Build history of the part. All positions in model axes, mm. A direction names the side the tool comes from. Give positions to 0.01 mm unless a question says otherwise; leave off trailing zeros. Answer as a JSON object with one key per item and string values. Group by question number.
Q1. Drop flat-ended pins along their axis: pin 1 (5 mm diameter, centred on x = -6.5, z = -1.5, fed in from +Y); pin 2 (5 mm diameter, centred on x = -4, z = -15.5, fed in from +Y); pin 3 (4 mm diameter, centred on x = -4.95, z = 4.95, fed in from -Y); pin 4 (1.8 mm diameter, centred on x = 10.45, z = -4, fed in from +Y). Give the stop position or say it passes through.
Q2. Wall check: probe 1 along X at (y, z) = (0.85, 4); probe 2 along Z at (x, y) = (6, 8.75); probe 3 along Z at (x, y) = (-6.25, 7.5). Give the ranges that are in metal, low to high. Write a range as from..to.
Q3. Two-plate mould, pull along X, no slides. Class faces 5 (the flat face through (8.5, 9, 0)), 6 (the cylindrical face through (0.13, 8.97, -13.25)), 7 (the cylindrical face through (-0.14, 10.49, -10.25)), 8 (the flat face through (0, 7, -20)): pulls with the +X half, pulls with the -X half, needs draft (parallel to the pull), parting line crosses it, or undercut.
Q4. Band-saw the part on A-A, the plane y = 1.25. Count the separate pieces of the cut face and the enclosed holes in it, plus the area to 3 significant figures.
Q5. Tool access for faces 1 (the cylindrical face through (-8.814, 4.163, -4.215)), 2 (the flat face through (-0.1, 11, -10.4)), 3 (the cylindrical face through (7.924, 4.327, -5.34)), 4 (the flat face through (-6.44, 1.01, -0.05)): list every direction of +Z, -Z, +X, -X, +Y, -Y with a clear straight run to the whole face (end or side of a thin tool).
from build123d import *

# Parameters (mm, degrees)
SKETCH1_W           = 25
SKETCH1_H           = 52
BOSS_EXTRUDE1_DEPTH = 7
SKETCH2_R           = 1
CUT_EXTRUDE1_DEPTH  = 30.685855218
LPATTERN1_COUNT     = 6
LPATTERN1_PITCH     = 8
CHAMFER2_SIZE       = 4
SKETCH10_W          = 14.9
SKETCH10_H          = 52
CUT_EXTRUDE4_DEPTH  = 2
CHAMFER3_SIZE       = 2
BOSS_EXTRUDE2_DEPTH = 3
BOSS_EXTRUDE3_DEPTH = 4
SKETCH13_R          = 1.65
CUT_EXTRUDE5_DEPTH  = 3
CUT_EXTRUDE6_REACH  = 31.686
SKETCH14_R          = 3
SKETCH16_R          = 1.65
CUT_EXTRUDE7_DEPTH  = 4.5


# Some blends are built 0.0001 mm under size
with BuildPart() as part:
    # Sketch1 → Boss-Extrude1 (new body)
    with BuildSketch(Plane(origin=(0, 0, 0), x_dir=(1, 0, 0), z_dir=(0, 1, 0))):
        Rectangle(SKETCH1_W, SKETCH1_H)
    extrude(amount=BOSS_EXTRUDE1_DEPTH)

    # Sketch2 → Cut-Extrude1 (cut, through all)
    with BuildSketch(Plane(origin=(0, 7, 0), x_dir=(1, 0, 0), z_dir=(0, 1, 0))):
        with Locations(Location((-10.45, -20, 0), (0, 0, 270))):
            Circle(SKETCH2_R)
        with Locations(Location((10.45, -20, 0), (0, 0, 270))):
            Circle(SKETCH2_R)
    cut_extrude1 = extrude(amount=-CUT_EXTRUDE1_DEPTH, mode=Mode.SUBTRACT)

    # LPattern1: Cut-Extrude1 ×6
    with Locations(*[(0, 0, -i * LPATTERN1_PITCH) for i in range(1, LPATTERN1_COUNT)]):
        add(cut_extrude1, mode=Mode.SUBTRACT)

    # Chamfer2
    # the kernel refuses this chamfer: 4 mm, written as the material it takes off along each edge
    with BuildSketch(Plane(origin=(-12.5, 7, -36.286731952), x_dir=(-0.027495876610586487, -0.9996219169112968, 0), z_dir=(0, 0, 1)), Plane(origin=(12.5, 7, 36.286731952), x_dir=(0.027495876610586487, -0.9996219169112968, 0), z_dir=(0, 0, -1))) as chamfer2_piece_1:
        Polygon((CHAMFER2_SIZE * 0.999621916911, CHAMFER2_SIZE * 0.0274958766106), (-CHAMFER2_SIZE * 0.0274958766106, CHAMFER2_SIZE * 0.999621916911), (0, 0), align=None)
    extrude(amount=72.573463904, mode=Mode.SUBTRACT)

    # Sketch10 → Cut-Extrude4 (cut)
    with BuildSketch(Plane.XZ):
        Rectangle(SKETCH10_W, SKETCH10_H)
    extrude(amount=-CUT_EXTRUDE4_DEPTH, mode=Mode.SUBTRACT)

    # Chamfer3
    chamfer3_edges = [part.edges().sort_by_distance(p)[0] for p in [
        (7.45, 2, 0),
        (-7.45, 2, 0),
    ]]
    chamfer(chamfer3_edges, length=CHAMFER3_SIZE - 0.0001)  # a hair under: the kernel refuses the full size

    # Sketch12 → Boss-Extrude2 (add)
    with BuildSketch(Plane(origin=(0, 7, 0), x_dir=(1, 0, 0), z_dir=(0, 1, 0))):
        with BuildLine():
            ThreePointArc((8.5, 5.728219619), (0, 10.25), (-8.5, 5.728219619))
            Line((-8.5, 5.728219619), (-8.5, -5.728219619))
            ThreePointArc((-8.5, -5.728219619), (0, -10.25), (8.5, -5.728219619))
            Line((8.5, -5.728219619), (8.5, 5.728219619))
        make_face()
    extrude(amount=BOSS_EXTRUDE2_DEPTH)

    # Sketch12<3> → Boss-Extrude3 (add)
    with BuildSketch(Plane(origin=(0, 7, 0), x_dir=(1, 0, 0), z_dir=(0, 1, 0))):
        with BuildLine():
            ThreePointArc((8.5, 10.164275675), (0, 13.25), (-8.5, 10.164275675))
            Line((-8.5, 10.164275675), (-8.5, 5.728219619))
            ThreePointArc((-8.5, 5.728219619), (0, 10.25), (8.5, 5.728219619))
            Line((8.5, 5.728219619), (8.5, 10.164275675))
        make_face()
        with BuildLine():
            Line((-8.5, -5.728219619), (-8.5, -10.164275675))
            ThreePointArc((-8.5, -10.164275675), (0, -13.25), (8.5, -10.164275675))
            Line((8.5, -10.164275675), (8.5, -5.728219619))
            ThreePointArc((8.5, -5.728219619), (0, -10.25), (-8.5, -5.728219619))
        make_face()
    extrude(amount=BOSS_EXTRUDE3_DEPTH)

    # Sketch13 → Cut-Extrude5 (cut)
    with BuildSketch(Plane(origin=(0, 10, 0), x_dir=(1, 0, 0), z_dir=(0, 1, 0))):
        with Locations(Location((-4.949747468, 4.949747468, 0), (0, 0, 270))):
            Circle(SKETCH13_R)
        with Locations(Location((4.949747468, 4.949747468, 0), (0, 0, 270))):
            Circle(SKETCH13_R)
        with Locations(Location((4.949747468, -4.949747468, 0), (0, 0, 270))):
            Circle(SKETCH13_R)
        with Locations(Location((-4.949747468, -4.949747468, 0), (0, 0, 270))):
            Circle(SKETCH13_R)
        with Locations(Location((0, 0, 0), (0, 0, 270))):
            Circle(SKETCH13_R)
    extrude(amount=-CUT_EXTRUDE5_DEPTH, mode=Mode.SUBTRACT)

    # Sketch14 → Cut-Extrude6 (cut, up to next)
    with BuildSketch(Plane(origin=(0, 7, 0), x_dir=(1, 0, 0), z_dir=(0, 1, 0)), mode=Mode.PRIVATE) as cut_extrude6_sk1:
        with Locations(Location((-4.949747468, 4.949747468, 0), (0, 0, 270))):
            Circle(SKETCH14_R)
    cut_extrude6_tool1 = extrude(cut_extrude6_sk1.sketch, amount=-CUT_EXTRUDE6_REACH, mode=Mode.PRIVATE) & part.part
    # Sketch14 → Cut-Extrude6 (cut, up to next)
    with BuildSketch(Plane(origin=(0, 7, 0), x_dir=(1, 0, 0), z_dir=(0, 1, 0)), mode=Mode.PRIVATE) as cut_extrude6_sk2:
        with Locations(Location((4.949747468, 4.949747468, 0), (0, 0, 270))):
            Circle(SKETCH14_R)
    cut_extrude6_tool2 = extrude(cut_extrude6_sk2.sketch, amount=-CUT_EXTRUDE6_REACH, mode=Mode.PRIVATE) & part.part
    # Sketch14 → Cut-Extrude6 (cut, up to next)
    with BuildSketch(Plane(origin=(0, 7, 0), x_dir=(1, 0, 0), z_dir=(0, 1, 0)), mode=Mode.PRIVATE) as cut_extrude6_sk3:
        with Locations(Location((4.949747468, -4.949747468, 0), (0, 0, 270))):
            Circle(SKETCH14_R)
    cut_extrude6_tool3 = extrude(cut_extrude6_sk3.sketch, amount=-CUT_EXTRUDE6_REACH, mode=Mode.PRIVATE) & part.part
    # Sketch14 → Cut-Extrude6 (cut, up to next)
    with BuildSketch(Plane(origin=(0, 7, 0), x_dir=(1, 0, 0), z_dir=(0, 1, 0)), mode=Mode.PRIVATE) as cut_extrude6_sk4:
        with Locations(Location((-4.949747468, -4.949747468, 0), (0, 0, 270))):
            Circle(SKETCH14_R)
    cut_extrude6_tool4 = extrude(cut_extrude6_sk4.sketch, amount=-CUT_EXTRUDE6_REACH, mode=Mode.PRIVATE) & part.part
    # Sketch14 → Cut-Extrude6 (cut, up to next)
    with BuildSketch(Plane(origin=(0, 7, 0), x_dir=(1, 0, 0), z_dir=(0, 1, 0)), mode=Mode.PRIVATE) as cut_extrude6_sk5:
        with Locations(Location((0, 0, 0), (0, 0, 270))):
            Circle(SKETCH14_R)
    cut_extrude6_tool5 = extrude(cut_extrude6_sk5.sketch, amount=-CUT_EXTRUDE6_REACH, mode=Mode.PRIVATE) & part.part
    add(cut_extrude6_tool1.solids().sort_by_distance((-4.949747, 7, -4.949747))[0], mode=Mode.SUBTRACT)
    add(cut_extrude6_tool2.solids().sort_by_distance((4.949747, 7, -4.949747))[0], mode=Mode.SUBTRACT)
    add(cut_extrude6_tool3.solids().sort_by_distance((4.949747, 7, 4.949747))[0], mode=Mode.SUBTRACT)
    add(cut_extrude6_tool4.solids().sort_by_distance((-4.949747, 7, 4.949747))[0], mode=Mode.SUBTRACT)
    add(cut_extrude6_tool5.solids().sort_by_distance((0, 7, 0))[0], mode=Mode.SUBTRACT)

    # Sketch16 → Cut-Extrude7 (cut)
    with BuildSketch(Plane(origin=(0, 7, 0), x_dir=(1, 0, 0), z_dir=(0, 1, 0))):
        with Locations(Location((-10.45, -20, 0), (0, 0, 270))):
            Circle(SKETCH16_R)
        with Locations(Location((10.45, -20, 0), (0, 0, 270))):
            Circle(SKETCH16_R)
        with Locations(Location((10.45, -12, 0), (0, 0, 270))):
            Circle(SKETCH16_R)
        with Locations(Location((-10.45, -12, 0), (0, 0, 270))):
            Circle(SKETCH16_R)
        with Locations(Location((10.45, -4, 0), (0, 0, 270))):
            Circle(SKETCH16_R)
        with Locations(Location((-10.45, -4, 0), (0, 0, 270))):
            Circle(SKETCH16_R)
        with Locations(Location((10.45, 4, 0), (0, 0, 270))):
            Circle(SKETCH16_R)
        with Locations(Location((-10.45, 4, 0), (0, 0, 270))):
            Circle(SKETCH16_R)
        with Locations(Location((10.45, 12, 0), (0, 0, 270))):
            Circle(SKETCH16_R)
        with Locations(Location((-10.45, 12, 0), (0, 0, 270))):
            Circle(SKETCH16_R)
        with Locations(Location((10.45, 20, 0), (0, 0, 270))):
            Circle(SKETCH16_R)
        with Locations(Location((-10.45, 20, 0), (0, 0, 270))):
            Circle(SKETCH16_R)
    extrude(amount=-CUT_EXTRUDE7_DEPTH, mode=Mode.SUBTRACT)


solid = part.part
Worked answers:
{
 "1": {"pin 1": "y = 10", "pin 2": "y = 7", "pin 3": "y = 7", "pin 4": "through"},
 "2": {"probe 1": "-12.5..-11.45, -9.45..-7.8, 7.8..9.45, 11.45..12.5", "probe 2": "-11.81..-6.22, -3.68..3.68, 6.22..11.81", "probe 3": "-11.68..-5.97, -3.93..3.93, 5.97..11.68"},
 "3": {"face 5": "pulls with the +X half", "face 6": "parting line crosses it", "face 7": "undercut", "face 8": "needs draft"},
 "4": {"separate pieces": "2", "enclosed holes": "12", "area": "590 mm2"},
 "5": {"face 1": "+Y", "face 2": "+Z, -Z, +X, -X, +Y", "face 3": "-Y", "face 4": "+Z, -Z, -Y"}
}
